The drawing under review shows one solid part. Ordinate dimensions are in mm from its lowest x, y, z. Round coordinates to 2 decimals unless told otherwise and drop trailing zeros. Order: outer loops, then holes, each group sorted by start corner. A loop starts at its lowest first (then second) coordinate and runs counter-clockwise, first axis right, second up. Notation, with made-up numbers: M 39,51.25 L 81,51.25 A19 cw 81,81.25 Z; hole C 39,58 d1. An arc over 180 degrees is marked long. Use a Markdown table: item, result.
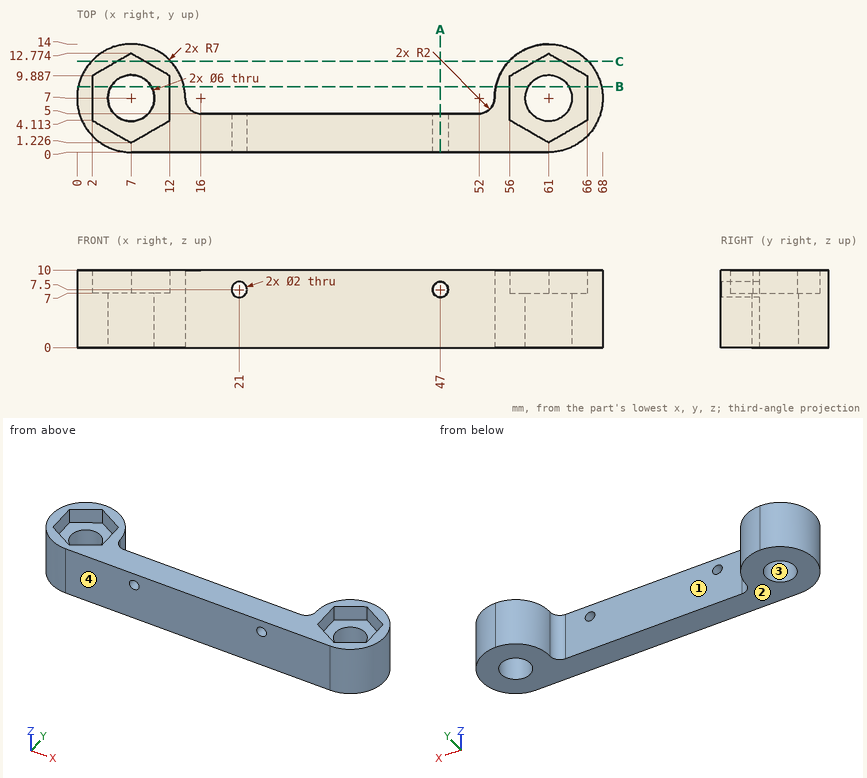
Q1. Add section B-B (y = 8.5). Write out the cut boundary in (x, z), then the cut area to 3 significant figures.
Determined:
| item | result |
|---|---|
| outline | M 0.16,0 L 4.4,0 L 4.4,7 L 2,7 L 2,10 L 0.16,10 Z; M 9.6,0 L 13.84,0 L 13.84,10 L 12,10 L 12,7 L 9.6,7 Z; M 54.16,0 L 58.4,0 L 58.4,7 L 56,7 L 56,10 L 54.16,10 Z; M 63.6,0 L 67.84,0 L 67.84,10 L 66,10 L 66,7 L 63.6,7 Z |
| area | 141 mm^2 |
Q2. Wall thickness on line 1 along X through (y, z) = (5.25, 3.25) (1 decimal); line 2 along Y through (x, z) = (46.5, 0.5); line 3 along Y through (x, z) = (60, 1.75): over which ranges is each line inside the solid? List them lowest first. Write a range as [from, to].
Determined:
| item | result |
|---|---|
| line 1 | x = [0.2, 4.6], [9.4, 15], [53, 58.6], [63.4, 67.8] |
| line 2 | y = [0, 5] |
| line 3 | y = [0, 4.17], [9.83, 13.93] |
Q3. Draft analysis for pull direction Y (two halves, no side actions). For the marked faces 1, 2, 3 and 4, state which applies: pulls with the +Y half, pulls with the -Y half, needs draft (parallel to the pull), parting line crosses it, or undercut.
Determined:
| item | result |
|---|---|
| face 1 | pulls with the +Y half |
| face 2 | needs draft |
| face 3 | undercut |
| face 4 | pulls with the -Y half |
Q4. Add section A-A (x = 47). Write out the cut boundary in (y, z).
Determined:
| item | result |
|---|---|
| outline | M 0,0 L 5,0 L 5,6.5 L 0,6.5 Z; M 0,8.5 L 5,8.5 L 5,10 L 0,10 Z |
Q5. Add section C-C (y = 11.75). Write out the cut boundary in (x, z).
Determined:
| item | result |
|---|---|
| outline | M 1.86,0 L 12.14,0 L 12.14,10 L 8.77,10 L 8.77,7 L 5.23,7 L 5.23,10 L 1.86,10 Z; M 55.86,0 L 66.14,0 L 66.14,10 L 62.77,10 L 62.77,7 L 59.23,7 L 59.23,10 L 55.86,10 Z |
Q6. Clearance check with flat-ended pins moving along their axes: pin 1 (3 mm diameter, centred on y = 2, z = 1, fed in from +X); pin 2 (1 mm diameter, centred on y = 2.5, z = 4.5, fed in from +X) (1 decimal); pin 3 (1.5 mm diameter, centred on y = 10, z = 7, fed in from +X); pin 4 (3.5 mm diameter, centred on x = 61, y = 7, fed in from -Z). State where each tip first meets the part, or that it passes through.
Determined:
| item | result |
|---|---|
| pin 1 | stops at x = 67.06 |
| pin 2 | stops at x = 66.7 |
| pin 3 | stops at x = 67.63 |
| pin 4 | passes through |
